Job drawing, mm, ordinate dimensions from the low corner. One solid piece. Round coordinates to 2 decimals unless told otherwise and drop trailing zeros. Loops run counter-clockwise (first coordinate to the right, second up) from the corner with the lowest first, then second, coordinate; pieces in that order, holes last.
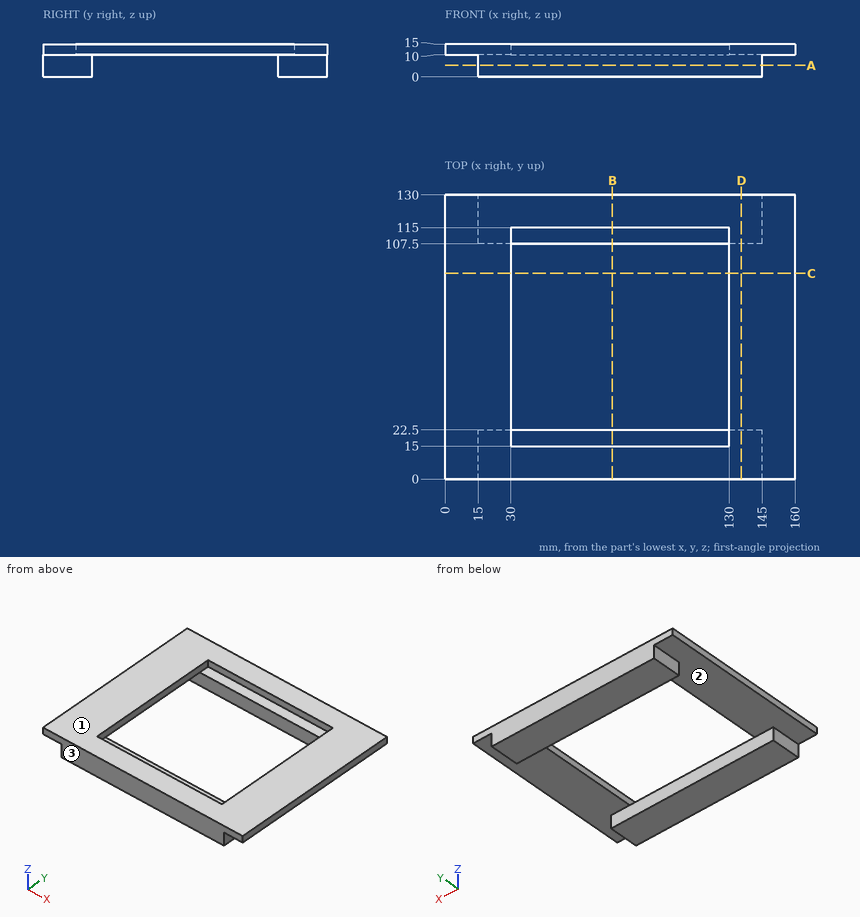
1) Slice it at D-D, the plane x = 135.5. Give the cut face in (y, z), then the cut area to 3 significant figures.
Values:
outline: (0, 0) - (22.5, 0) - (22.5, 10) - (107.5, 10) - (107.5, 0) - (130, 0) - (130, 15) - (0, 15) - close
area: 1,100 mm2
2) Slice it at B-B, the plane x = 76.5. Give the cut face in (y, z), then the cut area to 3 significant figures.
Values:
outline: (0, 0) - (22.5, 0) - (22.5, 10) - (15, 10) - (15, 15) - (0, 15) - close; (107.5, 0) - (130, 0) - (130, 15) - (115, 15) - (115, 10) - (107.5, 10) - close
area: 600 mm2
3) Drop flat-ended pins along their axis: pin 1 Ø3 at (y, z) = (9.5, 6) entering from -X; pin 2 Ø9 at (x, y) = (152, 95.5) entering from -Z; pin 3 Ø6 at (x, y) = (97, 111.5) entering from +Z. Give the stop position or say it passes through.
Values:
pin 1: stops at x = 15
pin 2: stops at z = 10
pin 3: stops at z = 10
4) Slice it at A-A, the plane z = 5.25. Give the cut face in (x, y), then the cut area to 3 significant figures.
Values:
outline: (15, 0) - (145, 0) - (145, 22.5) - (15, 22.5) - close; (15, 107.5) - (145, 107.5) - (145, 130) - (15, 130) - close
area: 5,850 mm2
5) Mould opens along Y. For the marked faces 1, 2 and 3 say: released by +Y, released by -Y, zero draft, split by the parting line, or undercut.
Values:
face 1: zero draft
face 2: undercut
face 3: released by -Y
6) Wall check: line 1 along Y through (x, z) = (104, 9.25); line 2 along X through (y, z) = (72, 12.75); line 3 along Y through (x, z) = (65.5, 12.5). Give the ranges that are in metal, low to high.
Values:
line 1: y = 0 to 22.5, 107.5 to 130
line 2: x = 0 to 30, 130 to 160
line 3: y = 0 to 15, 115 to 130
7) Slice it at C-C, the plane y = 94. Give the cut face in (x, z).
Values:
outline: (0, 10) - (30, 10) - (30, 15) - (0, 15) - close; (130, 10) - (160, 10) - (160, 15) - (130, 15) - close
